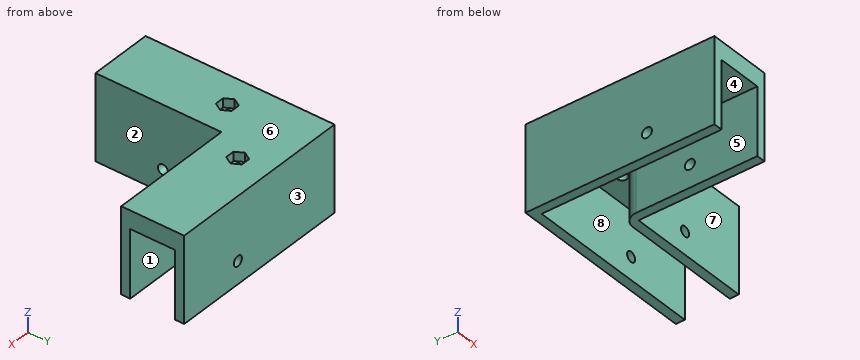
from build123d import *

# Parameters (mm, degrees)
BOSS_EXTRU_1_DEPTH      = 8
ENL_V_MAT_EXTRU_1_DEPTH = 4
ESQUISSE3_R             = 2.25
ENL_V_MAT_EXTRU_2_DEPTH = 5
BOSS_EXTRU_2_DEPTH      = 38
ESQUISSE5_R             = 2.25
ENL_V_MAT_EXTRU_3_DEPTH = 29
ESQUISSE6_R             = 2.25
ENL_V_MAT_EXTRU_4_DEPTH = 29
CONG_1_R                = 6


with BuildPart() as part:
    # Esquisse1 → Boss.-Extru.1 (new body)
    with BuildSketch(Plane.XY):
        Polygon((0, 0), (0, 60), (60, 60), (60, 80), (-20, 80), (-20, 0), align=None)
    extrude(amount=BOSS_EXTRU_1_DEPTH)

    # Esquisse2 → Enlèv. mat.-Extru.1 (cut)
    with BuildSketch(Plane.XY.offset(8)):
        Polygon((-14.041451884, 47.5), (-12.020725942, 51), (-7.979274058, 51), (-5.958548116, 47.5), (-7.979274058, 44), (-12.020725942, 44), align=None)
        Polygon((8.458548116, 70), (10.479274058, 73.5), (14.520725942, 73.5), (16.541451884, 70), (14.520725942, 66.5), (10.479274058, 66.5), align=None)
    extrude(amount=-ENL_V_MAT_EXTRU_1_DEPTH, mode=Mode.SUBTRACT)

    # Esquisse3 → Enlèv. mat.-Extru.2 (cut, through all)
    with BuildSketch(Plane.XY.offset(4)):
        with Locations((-10, 47.5)):
            Circle(ESQUISSE3_R)
        with Locations((12.5, 70)):
            Circle(ESQUISSE3_R)
    extrude(amount=-ENL_V_MAT_EXTRU_2_DEPTH, mode=Mode.SUBTRACT)

    # Esquisse4 → Boss.-Extru.2 (add)
    with BuildSketch(Plane.XY.offset(8)):
        Polygon((0, 0), (0, 60), (60, 60), (60, 56), (4, 56), (4, 0), align=None)
        Polygon((60, 80), (60, 84), (-24, 84), (-24, 0), (-20, 0), (-20, 80), align=None)
    extrude(amount=-BOSS_EXTRU_2_DEPTH)

    # Esquisse5 → Enlèv. mat.-Extru.3 (cut, through all)
    with BuildSketch(Plane.XZ.offset(-56)):
        with Locations((30, -20)):
            Circle(ESQUISSE5_R)
    extrude(amount=-ENL_V_MAT_EXTRU_3_DEPTH, mode=Mode.SUBTRACT)

    # Esquisse6 → Enlèv. mat.-Extru.4 (cut, through all)
    with BuildSketch(Plane(origin=(4, 0, 0), x_dir=(0, 0, -1), z_dir=(1, 0, 0))):
        with Locations(Location((20, 30, 0), (0, 0, 90))):  # turned: the seam where the file's is
            Circle(ESQUISSE6_R)
    extrude(amount=-ENL_V_MAT_EXTRU_4_DEPTH, mode=Mode.SUBTRACT)

    # Congé1
    cong_1_edges = [part.edges().sort_by_distance(p)[0] for p in [
        (0, 60, -15),
    ]]
    fillet(cong_1_edges, radius=CONG_1_R)


solid = part.part
For this review, take the finished solid that the model builds, in its own axes (mm). Face numbers are marked on the shaded views. A direction names the side the tool comes from. Coordinates: 2 decimals unless noted, no trailing zeros. Loops run counter-clockwise (first coordinate to the right, second up) from the corner with the lowest first, then second, coordinate; pieces in that order, holes last. Notation, with made-up numbers: (39, 41) - (96, 41) arc R9 cw to (96, 45) - close; hole circle Ø3 at (86, -35.75). An arc over 180 degrees is marked (long way). Use a Markdown table: item, result. Add a question column.
Item 1: Mouldability with a two-part tool opening along Y and no side actions: class the marked faces 6, 7 and 8 as pulls with the +Y half, pulls with the -Y half, needs draft (parallel to the pull), parting line crosses it, or undercut.
Item 2: We need section B-B (x = 30). Give the boundary of the cut face in (y, z), and give its area (3 significant figures).
Item 3: Insertion check: pin 1 Ø2.5 at (x, z) = (30, -20) entering from -Y; pin 2 Ø15 at (x, z) = (29, -20) entering from -Y; pin 3 Ø11.5 at (y, z) = (38, -11) entering from +X. Each pin has a flat end and moves straight along its axis. Give the tip position at first contact, or say it passes through.
Item 4: We need section D-D (z = -1.5). Give the boundary of the cut face in (x, y), and give its area (3 significant figures).
Item 5: We need section A-A (z = -20). Give the number of separate pieces and of enclosed holes in the cut face, and give its area (3 significant figures).
Item 6: Tool access review of the marked faces 1, 2, 3, 4 and 5: name each direction out of +Z, -Z, +X, -X, +Y, -Y from which nothing blocks a thin tool from reaching the whole face with its end or side.
Item 7: We need section C-C (y = 30). Give the boundary of the cut face in (x, z).
Item 8: For line 1 (X direction, y = 15, z = -19); line 2 (Y direction, x = 12.5, z = 1.95); line 3 (Z direction, x = 30, y = 58.55), list the stretches that pass through material, from the lowest coordinate up.
Results list:
| question | item | result |
|---|---|---|
| 1 | face 6 | needs draft |
| 1 | face 7 | pulls with the -Y half |
| 1 | face 8 | undercut |
| 2 | outline | (56, -30) - (60, -30) - (60, -22.25) - (56, -22.25) - close; (56, -17.75) - (60, -17.75) - (60, 0) - (80, 0) - (80, -17.75) - (84, -17.75) - (84, 8) - (56, 8) - close; (80, -30) - (84, -30) - (84, -22.25) - (80, -22.25) - close |
| 2 | area | 428 mm^2 |
| 3 | pin 1 | passes through |
| 3 | pin 2 | stops at y = 56 |
| 3 | pin 3 | stops at x = 4 |
| 4 | outline | (-24, 0) - (-20, 0) - (-20, 80) - (60, 80) - (60, 84) - (-24, 84) - close; (0, 0) - (4, 0) - (4, 56) - (60, 56) - (60, 60) - (6, 60) arc R6 ccw to (0, 54) - close |
| 4 | area | 1,110 mm^2 |
| 5 | separate pieces | 6 |
| 5 | enclosed holes | 0 |
| 5 | area | 1,040 mm^2 |
| 6 | face 1 | -Z, +X |
| 6 | face 2 | +Z, -Z, +X, -Y |
| 6 | face 3 | +Z, -Z, +X, -X, +Y |
| 6 | face 4 | -Z |
| 6 | face 5 | -Z, -Y |
| 7 | outline | (-24, -30) - (-20, -30) - (-20, -22.25) - (-24, -22.25) - close; (-24, -17.75) - (-20, -17.75) - (-20, 0) - (0, 0) - (0, -17.75) - (4, -17.75) - (4, 8) - (-24, 8) - close; (0, -30) - (4, -30) - (4, -22.25) - (0, -22.25) - close |
| 8 | line 1 | x = -24 to -20, 0 to 4 |
| 8 | line 2 | y = 56 to 67.75, 72.25 to 84 |
| 8 | line 3 | z = -30 to -22.25, -17.75 to 8 |
